Check sheet for the modelled part. Datum: model origin and axes. Units: mm. Face numbers are marked on the shaded views. A direction names the side the tool comes from. Coordinates: 2 decimals unless noted, no trailing zeros. Loops run counter-clockwise (first coordinate to the right, second up) from the corner with the lowest first, then second, coordinate; pieces in that order, holes last. Notation, with made-up numbers: M -2,33 L 10,33 A29 cw 10,53 Z; hole C 88,89 d9. An arc over 180 degrees is marked long. Use CSV: the item, a comma, the result in double quotes. Start each with the question number.
(1) Set-up check for the marked faces 4, 5 and 6: record each of +Z, -Z, +X, -X, +Y, -Y from which the full face is reachable in a straight line by a thin tool's end or side.
(2) Section check C-C on x = 4.5. Record the cut outline in (y, z).
(3) Scan lines: line 1 (X direction, y = 3, z = 7); line 2 (Y direction, x = 7.5, z = 5); line 3 (X direction, y = 3.4, z = 2.5). Record each from-to range of solid material in increasing order.
(4) Draft check along Y on the marked faces 1, 2 and 3. Enter one of: pulls with the +Y half, pulls with the -Y half, needs draft (parallel to the pull), parting line crosses it, or undercut.
(5) Section check A-A on y = 3. Record the cut outline in (x, z), and give its area (3 significant figures).
(6) Go/stop test with a flat-tipped pin: pin 1 Ø2 at (y, z) = (3, 5) entering from +X. Record where the tip stops, or that it passes through.
(7) Section check B-B on z = 3.25. Record the cut outline in (x, y), and give its area (3 significant figures).
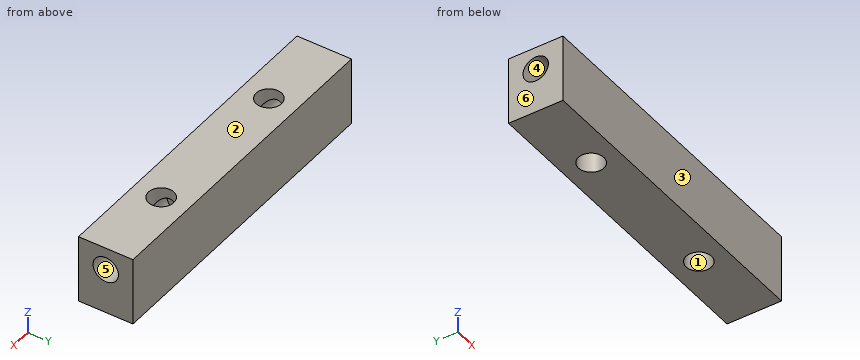
from build123d import *

# Parameters (mm, degrees)
F0_W     = 35.5
F0_H     = 6
F1_DEPTH = 7.5
F2_R     = 1.4
F3_DEPTH = 12
F4_R     = 1.4
F5_DEPTH = 12
F6_R     = 1.4
F7_DEPTH = 7.5


with BuildPart() as f1:
    # F0 (on Top) → F1 (new body)
    with BuildSketch(Plane.XY):
        with Locations((17.75, 3)):
            Rectangle(F0_W, F0_H)
    extrude(amount=F1_DEPTH)

    # F2 (on face) → F3 (cut)
    with BuildSketch(Plane.YZ.offset(35.5)):
        with Locations((3, 5)):
            Circle(F2_R)
    extrude(amount=-F3_DEPTH, mode=Mode.SUBTRACT)

    # F4 (on face) → F5 (cut)
    with BuildSketch(Plane(origin=(0, 0, 0), x_dir=(0, -1, 0), z_dir=(-1, 0, 0))):
        with Locations((-3, 5)):
            Circle(F4_R)
    extrude(amount=-F5_DEPTH, mode=Mode.SUBTRACT)

    # F6 (on face) → F7 (cut, through all)
    with BuildSketch(Plane(origin=(0, 0, 0), x_dir=(1, 0, 0), z_dir=(0, 0, -1))):
        with Locations((9, -3)):
            Circle(F6_R)
        with Locations((26.5, -3)):
            Circle(F6_R)
    extrude(amount=-F7_DEPTH, mode=Mode.SUBTRACT)


solid = f1.part
Outcome:
1,face 4,"-X"
1,face 5,"+X"
1,face 6,"+Z, -Z, -X, +Y, -Y"
2,outline,"M 0,0 L 6,0 L 6,7.5 L 0,7.5 Z; hole C 3,5 d2.8"
3,line 1,"x = 0 to 7.6, 10.4 to 25.1, 27.9 to 35.5"
3,line 2,"y = 0 to 1.6, 4.4 to 6"
3,line 3,"x = 0 to 7.66, 10.34 to 25.16, 27.84 to 35.5"
4,face 1,"undercut"
4,face 2,"needs draft"
4,face 3,"pulls with the -Y half"
5,outline,"M 0,0 L 7.6,0 L 7.6,3.6 L 0,3.6 Z; M 0,6.4 L 7.6,6.4 L 7.6,7.5 L 0,7.5 Z; M 10.4,0 L 25.1,0 L 25.1,3.6 L 23.5,3.6 L 23.5,6.4 L 25.1,6.4 L 25.1,7.5 L 10.4,7.5 L 10.4,6.4 L 12,6.4 L 12,3.6 L 10.4,3.6 Z; M 27.9,0 L 35.5,0 L 35.5,3.6 L 27.9,3.6 Z; M 27.9,6.4 L 35.5,6.4 L 35.5,7.5 L 27.9,7.5 Z"
5,area,"173 mm²"
6,pin 1,"stops at x = 23.5"
7,outline,"M 0,0 L 35.5,0 L 35.5,6 L 0,6 Z; hole C 9,3 d2.8; hole C 26.5,3 d2.8"
7,area,"201 mm²"
